Read the model definition and answer for the solid it produces. Units are mm, in the model's axes. Give positions to 0.01 mm unless a question says otherwise; leave off trailing zeros. Order: outer loops, then holes, each group sorted by start corner. A loop starts at its lowest first (then second) coordinate and runs counter-clockwise, first axis right, second up. Notation, with made-up numbers: (1.25, 10.5) - (9.25, 10.5) arc R9 ccw to (9.25, 24.5) - close; hole circle Ø5 at (68.5, 45.5). An arc over 180 degrees is marked (long way). Write item = value, one per line.
```python
from build123d import *

# Parameters (mm, degrees)
SKETCH1_R           = 68.659375
SKETCH1_R_2         = 55.959375
BOSS_EXTRUDE1_DEPTH = 3.175
BOSS_EXTRUDE2_START = -3.175
BOSS_EXTRUDE2_DEPTH = 3.175
CIRPATTERN1_COUNT   = 9


with BuildPart() as part:
    # Sketch1 → Boss-Extrude1 (new body)
    with BuildSketch(Plane(origin=(0, 0, 0), x_dir=(1, 0, 0), z_dir=(0, 1, 0))):
        with Locations(Location((0, 0, 0), (0, 0, 270))):
            Circle(SKETCH1_R)
        with Locations(Location((0, 0, 0), (0, 0, 270))):
            Circle(SKETCH1_R_2, mode=Mode.SUBTRACT)
    extrude(amount=BOSS_EXTRUDE1_DEPTH)

    # Sketch2 → Boss-Extrude2 (add)
    with BuildSketch(Plane(origin=(0, 3.175, 0), x_dir=(1, 0, 0), z_dir=(0, 1, 0)).offset(BOSS_EXTRUDE2_START)):
        with BuildLine():
            Line((-4.653697789, 71.001707707), (-5.372788209, 81.972907412))
            ThreePointArc((-5.372788209, 81.972907412), (0, 87.709375), (5.372788209, 81.972907412))
            ThreePointArc((5.372788209, 81.972907412), (1.580107525, 80.725221164), (0.983574692, 76.777399446))
            Line((0.983574692, 76.777399446), (3.889375, 69.933810414))
            ThreePointArc((3.889375, 69.933810414), (4.734169071, 68.871766239), (6.005193091, 68.39625305))
            ThreePointArc((6.005193091, 68.39625305), (-0.46538454, 68.657797755), (-6.931822104, 68.308561818))
            ThreePointArc((-6.931822104, 68.308561818), (-5.249012804, 69.195180628), (-4.653697789, 71.001707707))
        make_face()
    boss_extrude2 = extrude(amount=BOSS_EXTRUDE2_DEPTH)

    # CirPattern1: Boss-Extrude2 ×9 about axis
    cirpattern1_axis = Axis((0, 0, 0), (0, 1, 0))
    for i in range(1, CIRPATTERN1_COUNT):
        add(boss_extrude2.rotate(cirpattern1_axis, i * 360 / CIRPATTERN1_COUNT))


solid = part.part
```
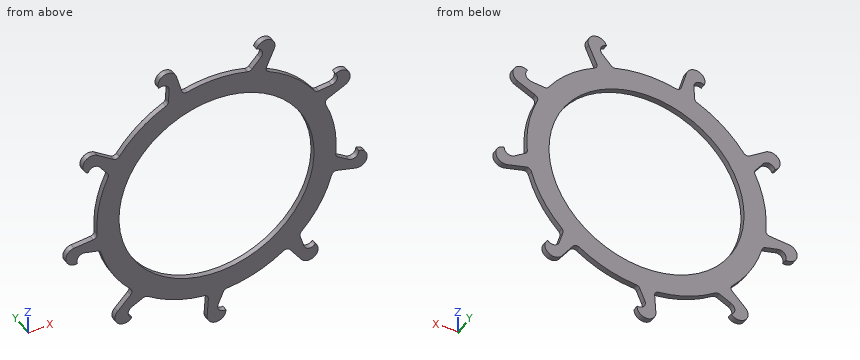
1. Flat-ended cylindrical pins translate along their axes: pin 1 (1.5 mm diameter, centred on x = -66, y = 1.5, fed in from +Z); pin 2 (2 mm diameter, centred on x = -57.5, z = -60.5, fed in from -Y); pin 3 (12 mm diameter, centred on x = -41, z = -63, fed in from +Y); pin 4 (1 mm diameter, centred on x = 17, y = 1.5, fed in from +Z). Find the tip coordinate at first contact, or state that the pin passes through.
Recorded:
pin_1 = 44.6
pin_2 = 0
pin_3 = through
pin_4 = 66.65
2. Straight lines are drawn through the part: L1, parallel to X at y = 0.2, z = 1.5; L2, parallel to X at y = 2.5, z = 0; L3, parallel to Z at x = -50, y = 1.7. For each, find the intervals that lie inside material, in ascending order. Write a range as [from, to].
Recorded:
L1 = [-68.64, -55.94], [55.94, 68.64]
L2 = [-68.66, -55.96], [55.96, 68.66]
L3 = [-67.59, -65.01], [-60.67, -52.23], [-47.05, -25.13], [25.13, 47.05]
3. Section A-A (z = 0) is taken. Determine the outline of the cut face in (x, y) (3 decimals).
Recorded:
outline = (-68.659, 0) - (-55.959, 0) - (-55.959, 3.175) - (-68.659, 3.175) - close; (55.959, 0) - (68.659, 0) - (68.659, 3.175) - (55.959, 3.175) - close
